Answer from the drawing. Dimensions are ordinates in mm from the lowest x, y and z of the part. A direction names the side the tool comes from. Round coordinates to 2 decimals unless told otherwise and drop trailing zeros. Loops run counter-clockwise (first coordinate to the right, second up) from the corner with the lowest first, then second, coordinate; pieces in that order, holes last. Notation, with made-up numbers: (59, 57) - (97, 57) arc R17 cw to (97, 62) - close; hole circle Ø6 at (48.5, -12.5). An arc over 180 degrees is marked (long way). Return JSON: item names as keys, results as strings.
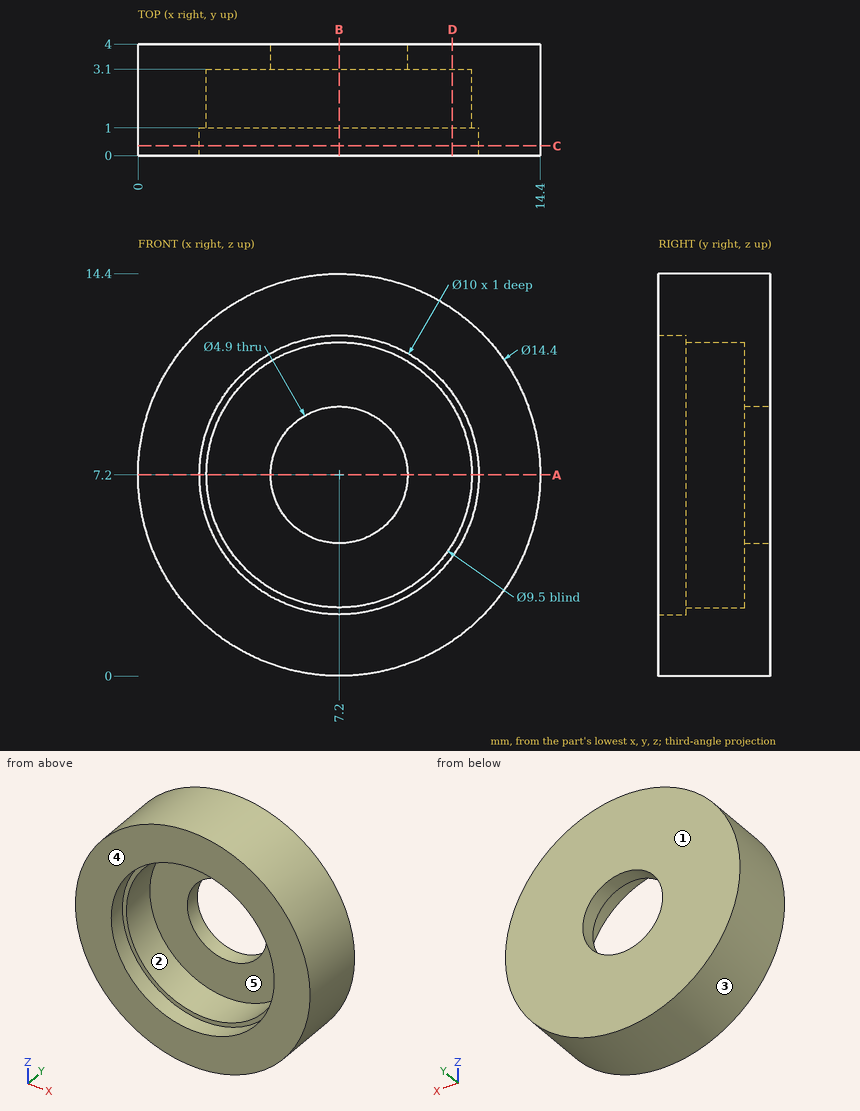
1) Section B-B (x = 7.2) is taken. Give the vertices of the cut face in (y, z).
Verdict:
{"outline": "(0, 0) - (4, 0) - (4, 4.75) - (3.1, 4.75) - (3.1, 2.45) - (1, 2.45) - (1, 2.2) - (0, 2.2) - close; (0, 12.2) - (1, 12.2) - (1, 11.95) - (3.1, 11.95) - (3.1, 9.65) - (4, 9.65) - (4, 14.4) - (0, 14.4) - close"}
2) Section C-C (y = 0.35) is taken. Give the vertices of the cut face in (x, z), and give its area (3 significant figures).
Verdict:
{"outline": "circle Ø14.4 at (7.2, 7.2); hole circle Ø10 at (7.2, 7.2)", "area": "84.3 mm2"}
3) Section A-A (z = 7.2) is taken. Give the vertices of the cut face in (x, y), and give its area (3 significant figures).
Verdict:
{"outline": "(0, 0) - (2.2, 0) - (2.2, 1) - (2.45, 1) - (2.45, 3.1) - (4.75, 3.1) - (4.75, 4) - (0, 4) - close; (9.65, 3.1) - (11.95, 3.1) - (11.95, 1) - (12.2, 1) - (12.2, 0) - (14.4, 0) - (14.4, 4) - (9.65, 4) - close", "area": "23.2 mm2"}
4) Find the intervals of material crossed by L1, parallel to Z at x = 7.2, y = 2.35; L2, parallel to Z at x = 7.2, y = 0.4; L3, parallel to Y at x = 8, z = 10, in increasing order.
Verdict:
{"L1": "z = 0 to 2.45, 11.95 to 14.4", "L2": "z = 0 to 2.2, 12.2 to 14.4", "L3": "y = 3.1 to 4"}
5) Flat-ended cylindrical pins translate along their axes: pin 1 (1.5 mm diameter, centred on y = 2, z = 1.5, fed in from -X); pin 2 (5 mm diameter, centred on x = 7, z = 8.5, fed in from -Y); pin 3 (1.5 mm diameter, centred on y = 2.5, z = 6, fed in from +X). Find the tip coordinate at first contact, or state that the pin passes through.
Verdict:
{"pin 1": "stops at x = 1.97", "pin 2": "stops at y = 3.1", "pin 3": "stops at x = 14.39"}
6) Determine the mould class of the marked faces 1, 2 and 3 for opening direction Z: pulls with the +Z half, pulls with the -Z half, needs draft (parallel to the pull), parting line crosses it, or undercut.
Verdict:
{"face 1": "needs draft", "face 2": "undercut", "face 3": "parting line crosses it"}
7) A tool of negligible diameter and unlimited length cuts with its end or side. For the marked faces 4 and 5, from which of +Z, -Z, +X, -X, +Y, -Y can it reach the whole face along a straight path? Write none if from no direction.
Verdict:
{"face 4": "+Z, -Z, +X, -X, -Y", "face 5": "-Y"}
8) Section D-D (x = 11.25) is taken. Give the vertices of the cut face in (y, z).
Verdict:
{"outline": "(0, 1.25) - (4, 1.25) - (4, 13.15) - (0, 13.15) - (0, 10.13) - (1, 10.13) - (1, 9.68) - (3.1, 9.68) - (3.1, 4.72) - (1, 4.72) - (1, 4.27) - (0, 4.27) - close"}
